Could you check a few things on this model? Use its own coordinates, in mm. A direction names the side the tool comes from. Give positions to 0.01 mm unless a question says otherwise; leave off trailing zeros. Order: outer loops, then holes, each group sorted by start corner. A loop starts at its lowest first (then second) coordinate and runs counter-clockwise, first axis right, second up. Notation, with made-up numbers: M 31,-36.75 L 71,-36.75 A20 ccw 71,-5.75 Z; hole C 82.5,79 d3. An arc over 180 degrees is marked long. Answer in a Markdown table with one row per item. Add a question column.
```python
from build123d import *

# Parameters (mm, degrees)
SKETCH_W        = 30
SKETCH_H        = 50
PAD_DEPTH       = 5
SKETCH002_W     = 30
SKETCH002_H     = 13
PAD001_DEPTH    = 11
GROOVE_ANGLE    = 180
SKETCH004_R     = 2.5
POCKET_DEPTH    = 4
SKETCH005_R     = 1.5
POCKET001_DEPTH = 5
SKETCH006_R     = 3.5
POCKET002_DEPTH = 3
SKETCH008_R     = 1.75
POCKET003_DEPTH = 3
SKETCH009_W     = 2
SKETCH009_H     = 6.5
PAD002_DEPTH    = 36.25
SKETCH010_W     = 6.5
SKETCH010_H     = 6.5
PAD003_DEPTH    = 3
SKETCH011_R     = 1.75
POCKET004_DEPTH = 3
SKETCH012_W     = 2
SKETCH012_H     = 6.5000000001
PAD004_DEPTH    = 36.25
SKETCH013_W     = 6.5
SKETCH013_H     = 6.5
PAD005_DEPTH    = 3
SKETCH014_R     = 1.75
POCKET005_DEPTH = 3
SKETCH015_W     = 2
SKETCH015_H     = 18.5
POCKET006_DEPTH = 5
SKETCH034_R     = 2.5
POCKET013_DEPTH = 3


with BuildPart() as part:
    # Sketch → Pad (new body)
    with BuildSketch(Plane.XY):
        with Locations((15, 25)):
            Rectangle(SKETCH_W, SKETCH_H)
    extrude(amount=PAD_DEPTH)

    # Sketch002 (on Face5 of Pad) → Pad001 (join)
    with BuildSketch(Plane(origin=(0, 0, 0), x_dir=(1, 0, 0), z_dir=(0, 0, -1))):
        with Locations((15, -6.5)):
            Rectangle(SKETCH002_W, SKETCH002_H)
    extrude(amount=PAD001_DEPTH)

    # Sketch003 (on Face10 of Pad001) → Groove (revolve, cut)
    with BuildSketch(Plane(origin=(0, 0, -11), x_dir=(1, 0, 0), z_dir=(0, 0, -1))):
        Polygon((7, -13), (7, -10.65), (8.97, -10.65), (8.97, -4.35), (7, -4.35), (7, 1), (15, 1), (15, -13), align=None)
    revolve(axis=Axis((15, -1, -11), (0, 1, 0)), revolution_arc=GROOVE_ANGLE, mode=Mode.SUBTRACT)

    # Sketch004 (on Face10 of Groove) → Pocket (cut)
    with BuildSketch(Plane(origin=(0, 0, -11), x_dir=(1, 0, 0), z_dir=(0, 0, -1))):
        with Locations((3.5, -6.5)):
            Circle(SKETCH004_R)
        with Locations((26.5, -6.5)):
            Circle(SKETCH004_R)
    extrude(amount=-POCKET_DEPTH, mode=Mode.SUBTRACT)

    # Sketch005 (on Face7 of Pocket) → Pocket001 (cut)
    with BuildSketch(Plane(origin=(0, 0, 0), x_dir=(1, 0, 0), z_dir=(0, 0, -1))):
        with Locations((10, -24)):
            Circle(SKETCH005_R)
        with Locations((20, -24)):
            Circle(SKETCH005_R)
        with Locations((10, -39)):
            Circle(SKETCH005_R)
        with Locations((20, -39)):
            Circle(SKETCH005_R)
    extrude(amount=-POCKET001_DEPTH, mode=Mode.SUBTRACT)

    # Sketch006 (on Face7 of Pocket001) → Pocket002 (cut)
    with BuildSketch(Plane(origin=(0, 0, 0), x_dir=(1, 0, 0), z_dir=(0, 0, -1))):
        with Locations((10, -39)):
            Circle(SKETCH006_R)
        with Locations((10, -24)):
            Circle(SKETCH006_R)
        with Locations((20, -24)):
            Circle(SKETCH006_R)
        with Locations((20, -39)):
            Circle(SKETCH006_R)
    extrude(amount=-POCKET002_DEPTH, mode=Mode.SUBTRACT)

    # Sketch008 (on Face8 of Pocket002) → Pocket003 (cut)
    with BuildSketch(Plane(origin=(0, 0, 0), x_dir=(0, -1, 0), z_dir=(-1, 0, 0))):
        with Locations((-3.25, 1.75)):
            Circle(SKETCH008_R)
    extrude(amount=-POCKET003_DEPTH, mode=Mode.SUBTRACT)

    # Sketch009 (on Face6 of Pocket003) → Pad002 (join)
    with BuildSketch(Plane(origin=(0, 0, 0), x_dir=(1, 0, 0), z_dir=(0, 0, -1))):
        with Locations((1, -38.25)):
            Rectangle(SKETCH009_W, SKETCH009_H)
    extrude(amount=PAD002_DEPTH)

    # Sketch010 (on Face21 of Pad002) → Pad003 (join)
    with BuildSketch(Plane.YZ.offset(2)):
        with Locations((38.25, -33)):
            Rectangle(SKETCH010_W, SKETCH010_H)
    extrude(amount=PAD003_DEPTH)

    # Sketch011 (on Face7 of Pad003) → Pocket004 (cut)
    with BuildSketch(Plane(origin=(0, 0, 0), x_dir=(0, -1, 0), z_dir=(-1, 0, 0))):
        with Locations((-38.25, -33)):
            Circle(SKETCH011_R)
    extrude(amount=-POCKET004_DEPTH, mode=Mode.SUBTRACT)

    # Sketch012 (on Face6 of Pocket004) → Pad004 (join)
    with BuildSketch(Plane(origin=(0, 0, 0), x_dir=(1, 0, 0), z_dir=(0, 0, -1))):
        with Locations((29, -38.25)):
            Rectangle(SKETCH012_W, SKETCH012_H)
    extrude(amount=PAD004_DEPTH)

    # Sketch013 (on Face21 of Pad004) → Pad005 (join)
    with BuildSketch(Plane(origin=(28, 0, 0), x_dir=(0, -1, 0), z_dir=(-1, 0, 0))):
        with Locations((-38.25, -33)):
            Rectangle(SKETCH013_W, SKETCH013_H)
    extrude(amount=PAD005_DEPTH)

    # Sketch014 (on Face12 of Pad005) → Pocket005 (cut)
    with BuildSketch(Plane.YZ.offset(30)):
        with Locations((38.25, -33)):
            Circle(SKETCH014_R)
        with Locations((3.25, 1.75)):
            Circle(SKETCH014_R)
    extrude(amount=-POCKET005_DEPTH, mode=Mode.SUBTRACT)

    # Sketch015 (on Face5 of Pocket005) → Pocket006 (cut)
    with BuildSketch(Plane.XY.offset(5)):
        with Locations((3, 31.5)):
            Rectangle(SKETCH015_W, SKETCH015_H)
        with Locations((27, 31.5)):
            Rectangle(SKETCH015_W, SKETCH015_H)
    extrude(amount=-POCKET006_DEPTH, mode=Mode.SUBTRACT)

    # Sketch034 (on Face5 of Pocket006) → Pocket013 (cut)
    with BuildSketch(Plane.XY.offset(5)):
        with Locations((3.767766953, 7.767766953)):
            Circle(SKETCH034_R)
        with Locations((26.232233047, 7.767766953)):
            Circle(SKETCH034_R)
    extrude(amount=-POCKET013_DEPTH, mode=Mode.SUBTRACT)


solid = part.part
```
1. For faces 1 (the flat face through (28, 38, -36.25)), 2 (the cylindrical face through (9.805, 22.513, 3.986)), 3 (the cylindrical face through (27.576, 9.876, 3.521)), 4 (the cylindrical face through (21.88, 21.05, 1.48)), 5 (the flat face through (27, 38, -33)), which set-ups out of +Z, -Z, +X, -X, +Y, -Y let a thin tool reach every point of the face, with its end or its side?
2. Thinking about a two-plate mould opening in Y: for faces 6 (the flat face through (24, 5, -11)), 7 (the flat face through (29, 41.5, -22)), 8 (the flat face through (3, 6, -7)), which applies, pulls with the +Y half, pulls with the -Y half, needs draft (parallel to the pull), parting line crosses it, or undercut?
3. Suppose I cut it at D-D on z = -9. List the corners of the cut face in (x, y) for me, plus the area to 3 significant figures.
4. Suppose I cut it at C-C on z = -2. List the corners of the cut face in (x, y) for me, plus the area to 3 significant figures.
5. Suppose I cut it at A-A on y = 31.5. List the corners of the cut face in (x, z) for me.
6. Will these pins go through, and if not, where does the flat tip stop? P1, Ø1, axis at x = 19, y = 41.5, coming from the -Z side; P2, Ø4, axis at x = 3.5, y = 6.5, coming from the -Z side; P3, Ø1, axis at y = 37.5, z = -33, coming from the +X side.
7. Suppose I cut it at B-B on z = -33. List the corners of the cut face in (x, y) for me, plus the area to 3 significant figures.
8. If I drill on line 1 along X through (y, z) = (24, 2.2); line 2 along Y through (x, z) = (10, 3.7); line 3 along Z through (x, y) = (0.7, 3.25), over which ranges is the centre line in solid material (lowest first)? Write a range as [from, to].
Findings below:
| question | item | result |
|---|---|---|
| 1 | face 1 | -Z, +X, -X, +Y, -Y |
| 1 | face 2 | +Z, -Z |
| 1 | face 3 | +Z |
| 1 | face 4 | -Z |
| 1 | face 5 | +X |
| 2 | face 6 | needs draft |
| 2 | face 7 | pulls with the +Y half |
| 2 | face 8 | undercut |
| 3 | outline | M 0,0 L 7.25,0 L 7.25,4.35 L 9.31,4.35 L 9.31,10.65 L 7.25,10.65 L 7.25,13 L 0,13 Z; M 0,35 L 2,35 L 2,41.5 L 0,41.5 Z; M 20.69,4.35 L 22.75,4.35 L 22.75,0 L 30,0 L 30,13 L 22.75,13 L 22.75,10.65 L 20.69,10.65 Z; M 28,35 L 30,35 L 30,41.5 L 28,41.5 Z; hole C 3.5,6.5 d5; hole C 26.5,6.5 d5 |
| 3 | area | 201 mm2 |
| 4 | outline | M 0,0 L 30,0 L 30,13 L 0,13 Z; M 0,35 L 2,35 L 2,41.5 L 0,41.5 Z; M 28,35 L 30,35 L 30,41.5 L 28,41.5 Z |
| 4 | area | 416 mm2 |
| 5 | outline | M 0,0 L 2,0 L 2,5 L 0,5 Z; M 4,0 L 26,0 L 26,5 L 4,5 Z; M 28,0 L 30,0 L 30,5 L 28,5 Z |
| 6 | P1 | z = 3 |
| 6 | P2 | z = -7 |
| 6 | P3 | x = 27 |
| 7 | outline | M 0,35 L 5,35 L 5,41.5 L 0,41.5 L 0,40 L 3,40 L 3,36.5 L 0,36.5 Z; M 25,35 L 30,35 L 30,36.5 L 27,36.5 L 27,40 L 30,40 L 30,41.5 L 25,41.5 Z |
| 7 | area | 44.0 mm2 |
| 8 | line 1 | [0, 2], [4, 6.5], [13.5, 16.5], [23.5, 26], [28, 30] |
| 8 | line 2 | [0, 22.5], [25.5, 37.5], [40.5, 50] |
| 8 | line 3 | [-11, 0], [3.5, 5] |
